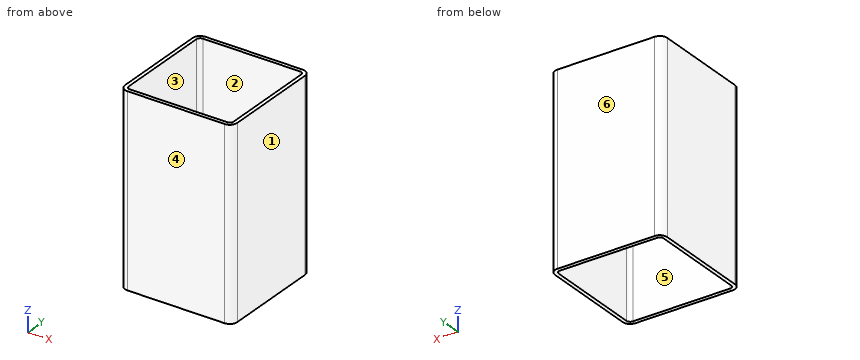
Autodesk Inventor part; units mm, degrees
ref_plane "Start plane" through (0, 0, 0) normal (0, 0, 1) x (1, 0, 0)
ref_plane "End plane" through (0, 0, 100) normal (0, 0, 1) x (1, 0, 0)
ref_plane "YZ Plane" through (0, 0, 0) normal (1, 0, 0) x (0, 1, 0)
ref_plane "Start plane" through (0, 0, 0) normal (0, 0, 1) x (1, 0, 0)
ref_plane "End plane" through (0, 0, 100) normal (0, 0, 1) x (1, 0, 0)
sketch "Sketch" plane through (0, 0, 0) normal (0, 0, 1) x (1, 0, 0)
  line L0 (-60, -52) -> (-60, 52)
  line L1 (-52, 60) -> (52, 60)
  line L2 (60, 52) -> (60, -52)
  line L3 (52, -60) -> (-52, -60)
  arc A0 (-60, -52) -> (-52, -60) centre (-52, -52) ccw
  arc A1 (-52, 60) -> (-60, 52) centre (-52, 52) ccw
  arc A2 (60, 52) -> (52, 60) centre (52, 52) ccw
  arc A3 (52, -60) -> (60, -52) centre (52, -52) ccw
  arc A4 (-52, 56) -> (-56, 52) centre (-52, 52) ccw
  line L4 (-52, 56) -> (52, 56)
  arc A5 (56, 52) -> (52, 56) centre (52, 52) ccw
  line L5 (56, 52) -> (56, -52)
  arc A6 (52, -56) -> (56, -52) centre (52, -52) ccw
  line L6 (52, -56) -> (-52, -56)
  arc A7 (-56, -52) -> (-52, -56) centre (-52, -52) ccw
  line L7 (-56, -52) -> (-56, 52)
  line L8 (0, 86.3196) -> (0, -86.3196) construction
  line L9 (-86.3196, 0) -> (86.3196, 0) construction
  circle A8 centre (0, 0) radius 4.9156 construction
  dimension "d7" = 8
  dimension "d10" = 120
  dimension "d11" = 120
  dimension "d12" = 4
  dimension "d15" = 60
  dimension "d16" = 60
extrude "Body" add sketch "Sketch" along normal blind 200
sketch "Sketch3" plane through (0, 0, 0) normal (0, 0, 1) x (1, 0, 0)
  line L0 (0, 0) -> (10, 0)
ref_plane "Work Plane3" through (0, 0, 0) normal (0, -1, 0) x (1, 0, 0)
sketch "Sketch4" plane through (0, 0, 0) normal (0, -1, 0) x (1, 0, 0)
  line L0 (-12.3242, 0) -> (13.7207, 0)
  line L1 (-12.3242, 100) -> (13.7207, 100)
  dimension "d18" = 100
sketch "Sketch5" plane through (0, 0, 0) normal (0, 0, 1) x (1, 0, 0)
  circle A0 centre (0, 0) radius 8.6035 construction
equation "\"d7\" = G_IR"
equation "\"d10\" = G_H"
equation "\"d11\" = G_W"
equation "\"d12\" = G_T"
equation "\"d15\" = 0.5 * d10"
equation "\"d16\" = 0.5 * d11"
equation "\"G_W\" = 120"
equation "\"G_H\" = 120"
equation "\"G_T\" = 4"
equation "\"G_IR\" = 8"
equation "\"G_L\" = d18"
equation "\"G_OFFSET_START\" = 0"
equation "\"G_OFFSET_END\" = 0"
properties part number "DIN EN 10219-2 - 120 x 120 x 4  - 100" material "Steel, Mild"
Build history of the part. All positions in model axes, mm. Face numbers are marked on the shaded views. A direction names the side the tool comes from. Coordinates: 2 decimals unless noted, no trailing zeros. Order: outer loops, then holes, each group sorted by start corner. A loop starts at its lowest first (then second) coordinate and runs counter-clockwise, first axis right, second up. Notation, with made-up numbers: M 18,14.25 L 66,14.25 A20 ccw 66,52.25 Z; hole C -36.5,55.25 d7. An arc over 180 degrees is marked long. One line per question, with ' | ' between items. Start each with the question number.
1. Wall check: line 1 along Y through (x, z) = (-51, 120); line 2 along Y through (x, z) = (-53, 105.5). Give the ranges that are in metal, low to high. Write a range as [from, to].
2. Mould opens along Y. For the marked faces 3, 4, 5 and 6 say: +Y half, -Y half, draft (parallel to the pull), parting line (faces both ways), or undercut.
3. Cut at A-A (x = -44). Write the cut outline in (y, z).
4. Tool access for the marked faces 1 and 2: list every direction of +Z, -Z, +X, -X, +Y, -Y with a clear straight run to the whole face (end or side of a thin tool).
5. Cut at B-B (z = 52.5). Write the cut outline in (x, y), plus the area to 3 significant figures.
The answers:
1) line 1: y = [-60, -56], [56, 60] | line 2: y = [-59.94, -55.87], [55.87, 59.94]
2) face 3: undercut | face 4: -Y half | face 5: undercut | face 6: +Y half
3) outline: M -60,0 L -56,0 L -56,200 L -60,200 Z; M 56,0 L 60,0 L 60,200 L 56,200 Z
4) face 1: +Z, -Z, +X, +Y, -Y | face 2: +Z, -Z
5) outline: M -60,-52 A8 ccw -52,-60 L 52,-60 A8 ccw 60,-52 L 60,52 A8 ccw 52,60 L -52,60 A8 ccw -60,52 Z; hole M -56,-52 A4 ccw -52,-56 L 52,-56 A4 ccw 56,-52 L 56,52 A4 ccw 52,56 L -52,56 A4 ccw -56,52 Z | area: 1,810 mm2
